For this review, take the finished solid that the model builds, in its own axes (mm). A direction names the side the tool comes from. Round coordinates to 2 decimals unless told otherwise and drop trailing zeros. Write each loop counter-clockwise with the first axis right and the second up, starting at its lowest first coordinate (ties: lowest second). Pieces come first, ordered by that corner, then holes. Notation, with made-up numbers: M 46.5,70 L 103.5,70 A20 ccw 103.5,86 Z; hole C 25,88 d9. An arc over 180 degrees is marked long. Use one line per item in the form item = value. Start each with the question number.
Item 1: Add section B-B (y = 2). State the section outline as (x, z) points, and give its area (3 significant figures).
Item 2: For faces 1 (the cylindrical face through (-1.48, 2.54, -0.69)), 2 (the flat face through (10.2, 3, 7)), 3 (the flat face through (16, 5.2, 11)), list the 3-axis set-ups (+Z, -Z, +X, -X, +Y, -Y) from which the entire face can be reached by the end or side of a thin tool; tool diameter is ignored.
Item 3: For line 1 (X direction, y = 0.75, z = 4.5); line 2 (Y direction, x = 26, z = 6); line 3 (Z direction, x = 28.5, y = 1), list the stretches that pass through material, from the lowest coordinate up. Write a range as [from, to].
Item 4: Add section D-D (z = 8.5). State the section outline as (x, y) points, and give its area (3 significant figures).
Item 5: Draft analysis for pull direction X (two halves, no side actions). For faces 4 (the cylindrical face through (16.35, -1.14, -1.1)), 5 (the flat face through (5, 3, 0)), 6 (the flat face through (-2, 3, 4)), state which applies: released by +X, released by -X, zero draft, split by the parting line, or undercut.
Item 6: For P1, Ø2.5, axis at x = 28, y = 1.5, coming from the +Z side; P2, Ø2, axis at x = 17, z = 12, coming from the -Y side; P3, Ø4, axis at x = 28.5, y = 1.5, coming from the +Z side, all flat-tipped, find the tip position at first contact; note any pin that passes through.
Item 7: Add section C-C (x = 3). State the section outline as (y, z) points.
Item 8: Add section A-A (z = 3.75). State the section outline as (x, y) points.
Autodesk Fusion 360 part; units mm, degrees
sketch "Sketch1" plane through (0, 0, 0) normal (0, 0, 1) x (1, 0, 0)
  line L0 (0, 0) -> (32.2, 0)
  line L1 (32.2, 0) -> (32.2, 5.2)
  line L2 (32.2, 5.2) -> (0, 5.2)
  line L3 (0, 5.2) -> (0, 0)
  line L4 (-2, -2) -> (34.2, -2)
  line L5 (34.2, -2) -> (34.2, 7.2)
  line L6 (34.2, 7.2) -> (-2, 7.2)
  line L7 (-2, 7.2) -> (-2, -2)
  line L8 (10.2, 5.2) -> (22, 5.2)
  line L9 (22, 5.2) -> (22, 0)
  line L10 (22, 0) -> (10.2, 0)
  line L11 (10.2, 0) -> (10.2, 5.2)
  dimension "d1" = 5.2
  dimension "d2" = 32.2
  dimension "d3" = 2
  dimension "d4" = 10.2
  dimension "d5" = 10.2
extrude "Extrude1" add sketch "Sketch1" along normal blind 8
extrude "Extrude2" add sketch "Sketch1" against normal blind 2 contours L0 L2 L3 L11 | L0 L2 L8 L9 L10 L11 | L0 L1 L2 L9 | L4 L5 L6 L7
extrude "Extrude3" add sketch "Sketch1" along normal blind 18 contours L0 L2 L8 L9 L10 L11
sketch "Sketch2" plane through (0, 5.2, 0) normal (0, 1, 0) x (-1, 0, 0)
  line L0 (-22, 8) -> (-10.2, 8)
  line L1 (-10.2, 8) -> (-10.2, 18)
  line L2 (-10.2, 18) -> (-22, 18)
  line L3 (-22, 18) -> (-22, 8)
  arc A0 (-22, 18) -> (-10.2, 18) centre (-16.1, 19.0909) ccw
  dimension "d19" = 6
extrude "Extrude4" cut sketch "Sketch2" against normal up to surface (5.2 mm away) contours L2 A0
fillet "Fillet1" radius 3 4 edges at (-2, 2.6, -2) (16.1, 7.2, -2) (34.2, 2.6, -2) (16.1, -2, -2)
fillet "Fillet3" radius 1 2 edges at (10.2, 2.6, 18) (22, 2.6, 18)
Calculated:
q1.outline = M -2,1 A3 ccw 1,-2 L 31.2,-2 A3 ccw 34.2,1 L 34.2,8 L 32.2,8 L 32.2,0 L 22,0 L 22,14.09 A1 ccw 20.3,14.81 A6 cw 11.9,14.81 A1 ccw 10.2,14.09 L 10.2,0 L 0,0 L 0,8 L -2,8 Z
q1.area = 266 mm^2
q2.face_1 = -Z, -X, +Y, -Y
q2.face_2 = +Z
q2.face_3 = +Z, +X, -X, +Y
q3.line_1 = [-2, 0], [10.2, 22], [32.2, 34.2]
q3.line_2 = [-2, 0], [5.2, 7.2]
q3.line_3 = [-2, 0]
q4.outline = M 10.2,0 L 22,0 L 22,5.2 L 10.2,5.2 Z
q4.area = 61.4 mm^2
q5.face_4 = zero draft
q5.face_5 = undercut
q5.face_6 = released by -X
q6.P1 = 0
q6.P2 = 0
q6.P3 = 8
q7.outline = M -2,1 A3 ccw 1,-2 L 4.2,-2 A3 ccw 7.2,1 L 7.2,8 L 5.2,8 L 5.2,0 L 0,0 L 0,8 L -2,8 Z
q8.outline = M -2,-2 L 34.2,-2 L 34.2,7.2 L -2,7.2 Z; hole M 0,0 L 10.2,0 L 10.2,5.2 L 0,5.2 Z; hole M 22,0 L 32.2,0 L 32.2,5.2 L 22,5.2 Z
